The listing builds one solid part. Answer for the finished solid, in the listing's coordinates (mm). A direction names the side the tool comes from. Coordinates: 2 decimals unless noted, no trailing zeros. Order: outer loops, then holes, each group sorted by start corner. A loop starts at its lowest first (then second) coordinate and runs counter-clockwise, first axis right, second up. Notation, with made-up numbers: (-33.5, 72) -> (3.5, 72) arc R21 ccw to (3.5, 93) -> close; hole circle Ø1 at (-27, 24.5). An arc over 180 degrees is marked (long way). Put each result on its own line as item: value. Start each with the question number.
```python
from build123d import *

# Parameters (mm, degrees)
SKETCH1_R             = 2.38125
BOSS_EXTRUDE1_DEPTH   = 5.298013245
SKETCH3_R             = 2.5
BOSS_EXTRUDE4_DEPTH   = 10
CHAMFER2_SIZE         = 1
FILLET1_R             = 2
CROQUIS1_R            = 2.5
CORTAR_EXTRUIR1_DEPTH = 10


with BuildPart() as part:
    # Sketch1 → Boss-Extrude1 (new body)
    with BuildSketch(Plane.XY):
        with BuildLine():
            Line((-13.245033113, 35.176307792), (-23.841059603, 29.058689045))
            ThreePointArc((-23.841059603, 29.058689045), (-33.537096789, 19.362651859), (-37.086092715, 6.117618746))
            Line((-37.086092715, 6.117618746), (-37.086092715, -6.117618746))
            ThreePointArc((-37.086092715, -6.117618746), (-33.537096789, -19.362651859), (-23.841059603, -29.058689045))
            Line((-23.841059603, -29.058689045), (-13.245033113, -35.176307792))
            ThreePointArc((-13.245033113, -35.176307792), (0, -38.725303718), (13.245033113, -35.176307792))
            Line((13.245033113, -35.176307792), (23.841059603, -29.058689045))
            ThreePointArc((23.841059603, -29.058689045), (33.537096789, -19.362651859), (37.086092715, -6.117618746))
            Line((37.086092715, -6.117618746), (37.086092715, 6.117618746))
            ThreePointArc((37.086092715, 6.117618746), (33.537096789, 19.362651859), (23.841059603, 29.058689045))
            Line((23.841059603, 29.058689045), (13.245033113, 35.176307792))
            ThreePointArc((13.245033113, 35.176307792), (0, 38.725303718), (-13.245033113, 35.176307792))
        make_face()
        with Locations((0, 31.78807947)):
            Circle(SKETCH1_R, mode=Mode.SUBTRACT)
        with Locations((27.529284359, 15.894039735)):
            Circle(SKETCH1_R, mode=Mode.SUBTRACT)
        with Locations((27.529284359, -15.894039735)):
            Circle(SKETCH1_R, mode=Mode.SUBTRACT)
        with Locations((0, -31.78807947)):
            Circle(SKETCH1_R, mode=Mode.SUBTRACT)
        with Locations((-27.529284359, -15.894039735)):
            Circle(SKETCH1_R, mode=Mode.SUBTRACT)
        with Locations((-27.529284359, 15.894039735)):
            Circle(SKETCH1_R, mode=Mode.SUBTRACT)
    extrude(amount=BOSS_EXTRUDE1_DEPTH)

    # Sketch3 → Boss-Extrude4 (add)
    with BuildSketch(Plane.XY.offset(5.298013245)):
        with BuildLine():
            Line((-2.5, 16.909480566), (-13.394039735, 10.619803793))
            ThreePointArc((-13.394039735, 10.619803793), (-15.224166754, 8.789676774), (-15.894039735, 6.289676774))
            Line((-15.894039735, 6.289676774), (-15.894039735, -6.289676774))
            ThreePointArc((-15.894039735, -6.289676774), (-15.224166754, -8.789676774), (-13.394039735, -10.619803793))
            Line((-13.394039735, -10.619803793), (-2.5, -16.909480566))
            ThreePointArc((-2.5, -16.909480566), (0, -17.579353547), (2.5, -16.909480566))
            Line((2.5, -16.909480566), (13.394039735, -10.619803793))
            ThreePointArc((13.394039735, -10.619803793), (15.224166754, -8.789676774), (15.894039735, -6.289676774))
            Line((15.894039735, -6.289676774), (15.894039735, 6.289676774))
            ThreePointArc((15.894039735, 6.289676774), (15.224166754, 8.789676774), (13.394039735, 10.619803793))
            Line((13.394039735, 10.619803793), (2.5, 16.909480566))
            ThreePointArc((2.5, 16.909480566), (0, 17.579353547), (-2.5, 16.909480566))
        make_face()
        Circle(SKETCH3_R, mode=Mode.SUBTRACT)
    extrude(amount=BOSS_EXTRUDE4_DEPTH)

    # Chamfer2
    chamfer2_edges = [part.edges().sort_by_distance(p)[0] for p in [
        (15.224166754, 8.789676774, 5.298013245),
        (7.947019868, 13.764642179, 5.298013245),
        (0, 17.579353547, 5.298013245),
        (-7.947019868, 13.764642179, 5.298013245),
        (-15.224166754, 8.789676774, 5.298013245),
        (-15.894039735, 0, 5.298013245),
        (-15.224166754, -8.789676774, 5.298013245),
        (-7.947019868, -13.764642179, 5.298013245),
        (0, -17.579353547, 5.298013245),
        (7.947019868, -13.764642179, 5.298013245),
        (15.224166754, -8.789676774, 5.298013245),
        (15.894039735, 0, 5.298013245),
    ]]
    chamfer(chamfer2_edges, length=CHAMFER2_SIZE)

    # Fillet1
    fillet1_edges = [part.edges().sort_by_distance(p)[0] for p in [
        (15.224166754, 8.789676774, 15.298013245),
        (7.947019868, 13.764642179, 15.298013245),
        (0, 17.579353547, 15.298013245),
        (-7.947019868, 13.764642179, 15.298013245),
        (-15.224166754, 8.789676774, 15.298013245),
        (-15.894039735, 0, 15.298013245),
        (-15.224166754, -8.789676774, 15.298013245),
        (-7.947019868, -13.764642179, 15.298013245),
        (0, -17.579353547, 15.298013245),
        (7.947019868, -13.764642179, 15.298013245),
        (15.224166754, -8.789676774, 15.298013245),
        (15.894039735, 0, 15.298013245),
    ]]
    fillet(fillet1_edges, radius=FILLET1_R)

    # Croquis1 → Cortar-Extruir1 (cut)
    with BuildSketch(Plane.XY.offset(5.298013245)):
        Circle(CROQUIS1_R)
    extrude(amount=-CORTAR_EXTRUIR1_DEPTH, mode=Mode.SUBTRACT)


solid = part.part
```
(1) The part is cut by section C-C on z = 14.25. Determine the outline of the cut face in (x, y).
(2) For a pull along X with two mould halves and no side action, classify faces 1 (the cylindrical face through (-25.258, -15.179, 2.612)), 2 (the cylindrical face through (-0.194, -38.725, 2.612)), 3 (the flat face through (15.894, 0, 10)) as released by +X, released by -X, zero draft, split by the parting line, or undercut.
(3) The part is cut by section B-B on x = 0. Determine the outline of the cut face in (y, z), plus the area to 3 significant figures.
(4) The part is cut by section A-A on y = 0. Determine the outline of the cut face in (x, z).
(5) Find the intervals of material crossed by L1, parallel to Y at x = 0, z = 4.2; L2, parallel to Y at x = 27.5, z = 4.5; L3, parallel to X at y = 18, z = 3.75, in increasing order.
(6) The part is cut by section D-D on z = 1. Determine the outline of the cut face in (x, y).
(7) Each of these flat-tipped pins is pushed along its axis until it touches: P1, Ø5.5, axis at y = 2, z = 11.5, coming from the +X side; P2, Ø5, axis at y = -15.5, z = 9.5, coming from the -X side; P3, Ø7.5, axis at y = 1.5, z = 11, coming from the -X side. Where does it stop, or does it pass through?
(8) A tool of negligible diameter and unlimited length cuts with its end or side. For faces 4 (the cylindrical face through (-0.04, -17.58, 9.75)), 5 (the cylindrical face through (0.04, 17.58, 9.75)), 6 (the flat face through (7.87, -13.81, 9.75)), 7 (the cylindrical face through (-7.738, 13.227, 14.697)), 8 (the flat face through (-17, 9, 5.298)), from which of +Z, -Z, +X, -X, +Y, -Y can it reach the whole face along a straight path? Write none if from no direction.
Worked out:
1. outline: (-15.65, -6.29) arc R4.76 ccw to (-13.27, -10.41) -> (-2.38, -16.7) arc R4.76 ccw to (2.38, -16.7) -> (13.27, -10.41) arc R4.76 ccw to (15.65, -6.29) -> (15.65, 6.29) arc R4.76 ccw to (13.27, 10.41) -> (2.38, 16.7) arc R4.76 ccw to (-2.38, 16.7) -> (-13.27, 10.41) arc R4.76 ccw to (-15.65, 6.29) -> close; hole circle Ø5 at (0, 0)
2. face 1: undercut
2. face 2: split by the parting line
2. face 3: released by +X
3. outline: (-38.73, 0) -> (-34.17, 0) -> (-34.17, 5.3) -> (-38.73, 5.3) -> close; (-29.41, 0) -> (-2.5, 0) -> (-2.5, 15.3) -> (-15.58, 15.3) arc R2 ccw to (-17.58, 13.3) -> (-17.58, 6.3) -> (-18.58, 5.3) -> (-29.41, 5.3) -> close; (2.5, 0) -> (29.41, 0) -> (29.41, 5.3) -> (18.58, 5.3) -> (17.58, 6.3) -> (17.58, 13.3) arc R2 ccw to (15.58, 15.3) -> (2.5, 15.3) -> close; (34.17, 0) -> (38.73, 0) -> (38.73, 5.3) -> (34.17, 5.3) -> close
3. area: 634 mm2
4. outline: (-37.09, 0) -> (-2.5, 0) -> (-2.5, 15.3) -> (-13.89, 15.3) arc R2 ccw to (-15.89, 13.3) -> (-15.89, 6.3) -> (-16.89, 5.3) -> (-37.09, 5.3) -> close; (2.5, 0) -> (37.09, 0) -> (37.09, 5.3) -> (16.89, 5.3) -> (15.89, 6.3) -> (15.89, 13.3) arc R2 ccw to (13.89, 15.3) -> (2.5, 15.3) -> close
5. L1: -38.73 to -34.17, -29.41 to -2.5, 2.5 to 29.41, 34.17 to 38.73
5. L2: -26.51 to -18.28, -13.51 to 13.51, 18.28 to 26.51
5. L3: -34.27 to -28.64, -26.42 to 26.42, 28.64 to 34.27
6. outline: (-37.09, -6.12) arc R26.49 ccw to (-23.84, -29.06) -> (-13.25, -35.18) arc R26.49 ccw to (13.25, -35.18) -> (23.84, -29.06) arc R26.49 ccw to (37.09, -6.12) -> (37.09, 6.12) arc R26.49 ccw to (23.84, 29.06) -> (13.25, 35.18) arc R26.49 ccw to (-13.25, 35.18) -> (-23.84, 29.06) arc R26.49 ccw to (-37.09, 6.12) -> close; hole circle Ø4.76 at (-27.53, -15.89); hole circle Ø4.76 at (-27.53, 15.89); hole circle Ø5 at (0, 0); hole circle Ø4.76 at (0, -31.79); hole circle Ø4.76 at (0, 31.79); hole circle Ø4.76 at (27.53, -15.89); hole circle Ø4.76 at (27.53, 15.89)
7. P1: x = 15.89
7. P2: x = -9.27
7. P3: x = -15.89
8. face 4: +Z, -Y
8. face 5: +Z, +Y
8. face 6: +Z, +X, -Y
8. face 7: +Z, -X, +Y
8. face 8: +Z
